Here's how the part is built. I have some questions about the finished solid (model axes, mm). Coordinates: 2 decimals unless noted, no trailing zeros. Write each loop counter-clockwise with the first axis right and the second up, starting at its lowest first coordinate (ties: lowest second). Pieces come first, ordered by that corner, then holes. Notation, with made-up numbers: (-3, 47) -> (13, 47) arc R16 ccw to (13, 64) -> close; hole circle Ø3 at (57, -21.5). An arc over 180 degrees is marked (long way). Put each result on its own line as item: value.
```python
from build123d import *

# Parameters (mm, degrees)
F0_W     = 254
F0_H     = 254
F1_DEPTH = 127
F2_R     = 12.7
F3_R     = 50.8
F4_DEPTH = 254.001
F5_R     = 5.08


with BuildPart() as f1:
    # F0 (on Front) → F1 (new body, symmetric)
    with BuildSketch(Plane.XZ):
        Rectangle(F0_W, F0_H)
    extrude(amount=F1_DEPTH, both=True)

    # F2
    f2_edges = [f1.edges().sort_by_distance(p)[0] for p in [
        (127, -127, 0),
        (0, -127, 127),
        (-127, -127, 0),
        (0, -127, -127),
        (-127, 0, 127),
        (-127, 127, 0),
        (-127, 0, -127),
        (127, 0, 127),
        (0, 127, 127),
        (127, 127, 0),
        (0, 127, -127),
        (127, 0, -127),
    ]]
    fillet(f2_edges, radius=F2_R)

    # F3 (on face) → F4 (cut, through all)
    with BuildSketch(Plane(origin=(0, 127, 0), x_dir=(-1, 0, 0), z_dir=(0, 1, 0))):
        Circle(F3_R)
    extrude(amount=-F4_DEPTH, mode=Mode.SUBTRACT)

    # F5
    f5_edges = [f1.edges().sort_by_distance(p)[0] for p in [
        (50.8, 127, 0),
        (50.8, -127, 0),
    ]]
    fillet(f5_edges, radius=F5_R)


solid = f1.part
```
Item 1: Imagine slicing it at B-B on y = -103.5. Write out the boundary of the cut face in (x, z).
Output:
outline: (-127, -114.3) arc R12.7 ccw to (-114.3, -127) -> (114.3, -127) arc R12.7 ccw to (127, -114.3) -> (127, 114.3) arc R12.7 ccw to (114.3, 127) -> (-114.3, 127) arc R12.7 ccw to (-127, 114.3) -> close; hole circle Ø101.6 at (0, 0)
Item 2: Imagine slicing it at A-A on x = 0. Write out the boundary of the cut face in (y, z), then the cut area to 3 significant figures.
Output:
outline: (-127, -114.3) arc R12.7 ccw to (-114.3, -127) -> (114.3, -127) arc R12.7 ccw to (127, -114.3) -> (127, -55.88) arc R5.08 ccw to (121.92, -50.8) -> (-121.92, -50.8) arc R5.08 ccw to (-127, -55.88) -> close; (-127, 55.88) arc R5.08 ccw to (-121.92, 50.8) -> (121.92, 50.8) arc R5.08 ccw to (127, 55.88) -> (127, 114.3) arc R12.7 ccw to (114.3, 127) -> (-114.3, 127) arc R12.7 ccw to (-127, 114.3) -> close
area: 38,500 mm²
Item 3: Please list where these lines run through material, in increasing order: line 1 along Z through (x, y) = (-1, 34.5); line 2 along Z through (x, y) = (-10, -2); line 3 along X through (y, z) = (56.5, -38.5). Write a range as from..to.
Output:
line 1: z = -127..-50.79, 50.79..127
line 2: z = -127..-49.81, 49.81..127
line 3: x = -127..-33.14, 33.14..127
Item 4: Imagine slicing it at C-C on z = 0. Write out the boundary of the cut face in (x, y).
Output:
outline: (-127, -114.3) arc R12.7 ccw to (-114.3, -127) -> (-55.88, -127) arc R5.08 ccw to (-50.8, -121.92) -> (-50.8, 121.92) arc R5.08 ccw to (-55.88, 127) -> (-114.3, 127) arc R12.7 ccw to (-127, 114.3) -> close; (50.8, -121.92) arc R5.08 ccw to (55.88, -127) -> (114.3, -127) arc R12.7 ccw to (127, -114.3) -> (127, 114.3) arc R12.7 ccw to (114.3, 127) -> (55.88, 127) arc R5.08 ccw to (50.8, 121.92) -> close
Item 5: If we mould it in two halves opening along X, with no side actions, what happens to faces 1 (the flat face through (-52, 127, 27)), 2 (the cylindrical face through (11.012, 1.707, -49.592)), 3 (the flat face through (-127, -2, -2))? For each: released by +X, released by -X, zero draft, split by the parting line, or undercut.
Output:
face 1: zero draft
face 2: undercut
face 3: released by -X
